```python
from build123d import *

# Parameters (mm, degrees)
SKETCH5_W           = 31
SKETCH5_H           = 31
BOSS_EXTRUDE2_DEPTH = 50
SKETCH6_W           = 5
SKETCH6_H           = 16
CUT_EXTRUDE1_DEPTH  = 50
CIRPATTERN1_COUNT   = 4
SKETCH7_R           = 5.164102758
CUT_EXTRUDE2_DEPTH  = 50
CIRPATTERN2_COUNT   = 4
FILLET1_R           = 1.5
SKETCH8_R           = 4.25
CUT_EXTRUDE3_DEPTH  = 1.5


with BuildPart() as part:
    # Sketch5 → Boss-Extrude2 (new body)
    with BuildSketch(Plane(origin=(0, 3, 0), x_dir=(1, 0, 0), z_dir=(0, 1, 0))):
        Rectangle(SKETCH5_W, SKETCH5_H)
    extrude(amount=BOSS_EXTRUDE2_DEPTH)

    # Sketch6 → Cut-Extrude1 (cut)
    with BuildSketch(Plane(origin=(0, 53, 0), x_dir=(1, 0, 0), z_dir=(0, 1, 0))):
        with Locations((-13, 0)):
            Rectangle(SKETCH6_W, SKETCH6_H)
    cut_extrude1 = extrude(amount=-CUT_EXTRUDE1_DEPTH, mode=Mode.SUBTRACT)

    # CirPattern1: Cut-Extrude1 ×4 about axis
    cirpattern1_axis = Axis((0, 0, 0), (0, 1, 0))
    for i in range(1, CIRPATTERN1_COUNT):
        add(cut_extrude1.rotate(cirpattern1_axis, i * 360 / CIRPATTERN1_COUNT), mode=Mode.SUBTRACT)

    # Sketch7 → Cut-Extrude2 (cut)
    with BuildSketch(Plane(origin=(0, 53, 0), x_dir=(1, 0, 0), z_dir=(0, 1, 0))):
        with Locations((-15.5, -15.5)):
            Circle(SKETCH7_R)
    cut_extrude2 = extrude(amount=-CUT_EXTRUDE2_DEPTH, mode=Mode.SUBTRACT)

    # CirPattern2: Cut-Extrude2 ×4 about axis
    cirpattern2_axis = Axis((0, 0, 0), (0, 1, 0))
    for i in range(1, CIRPATTERN2_COUNT):
        add(cut_extrude2.rotate(cirpattern2_axis, i * 360 / CIRPATTERN2_COUNT), mode=Mode.SUBTRACT)

    # Fillet1
    fillet1_edges = [part.edges().sort_by_distance(p)[0] for p in [
        (15.5, 28, -10.335897242),
        (10.335897242, 28, -15.5),
        (-10.335897242, 28, -15.5),
        (-15.5, 28, -10.335897242),
        (-15.5, 28, 10.335897242),
        (-10.335897242, 28, 15.5),
        (10.335897242, 28, 15.5),
        (15.5, 28, 10.335897242),
    ]]
    fillet(fillet1_edges, radius=FILLET1_R)

    # Sketch8 → Cut-Extrude3 (cut)
    with BuildSketch(Plane.XZ.offset(-3)):
        with Locations(Location((0, 0, 0), (0, 0, 270))):
            Circle(SKETCH8_R)
    extrude(amount=-CUT_EXTRUDE3_DEPTH, mode=Mode.SUBTRACT)


solid = part.part
```
Check sheet for the modelled part. Datum: model origin and axes. Units: mm. A direction names the side the tool comes from. Give positions to 0.01 mm unless a question says otherwise; leave off trailing zeros. Loops run counter-clockwise (first coordinate to the right, second up) from the corner with the lowest first, then second, coordinate; pieces in that order, holes last. Notation, with made-up numbers: M -32.5,20.5 L 1.5,20.5 A24 cw 1.5,31.5 Z; hole C 85,29 d9. An arc over 180 degrees is marked long. Answer in a Markdown table with one row per item.
1) Mould release check, pull along X, two halves, no side actions. Record for faces 1 (the face through (0, 28, -10.5)), 2 (the face through (15.5, 27.6, 8.5)), 3 (the face through (-15.18, 27.65, -9.93)), 4 (the face through (-13, 28, -8)): released by +X, released by -X, zero draft, split by the parting line, or undercut.
Solutions:
| item | result |
|---|---|
| face 1 | undercut |
| face 2 | released by +X |
| face 3 | released by -X |
| face 4 | zero draft |
2) Cross-section at B-B (z = 13.5). Enter the section's corners in (x, y).
Solutions:
| item | result |
|---|---|
| outline | M -10.74,3 L -8,3 L -8,53 L -10.74,53 Z; M 8,3 L 10.74,3 L 10.74,53 L 8,53 Z |
3) Depth check by flat-ended pin: pin 1 (1.5 mm diameter, centred on x = 12, y = 24.5, fed in from +Z); pin 2 (1.5 mm diameter, centred on x = 14, y = 19, fed in from -Z); pin 3 (5 mm diameter, centred on y = 16, z = -1.5, fed in from +X). Enter the tip coordinate at first touch or a pass-through.
Solutions:
| item | result |
|---|---|
| pin 1 | stops at z = 12.57 |
| pin 2 | stops at z = -10.85 |
| pin 3 | stops at x = 10.5 |
4) Cross-section at A-A (x = 0). Enter the section's corners in (y, z).
Solutions:
| item | result |
|---|---|
| outline | M 3,-10.5 L 53,-10.5 L 53,10.5 L 3,10.5 L 3,4.25 L 4.5,4.25 L 4.5,-4.25 L 3,-4.25 Z |
5) Thickness scan on line 1 (X direction, y = 3.75, z = 0); line 2 (X direction, y = 31, z = -7.5); line 3 (X direction, y = 36.5, z = 11.5). Record the ranges inside material, lowest first.
Solutions:
| item | result |
|---|---|
| line 1 | x = -10.5 to -4.25, 4.25 to 10.5 |
| line 2 | x = -10.5 to 10.5 |
| line 3 | x = -12.23 to -8, 8 to 12.23 |
6) Tool access check on faces 5 (the face through (-8, 28, -13)), 6 (the face through (0, 4.5, 0)), 7 (the face through (10.5, 28, 0)). Record the directions out of +Z, -Z, +X, -X, +Y, -Y that give a thin tool (end or side, any length) a straight path to the whole face; none if there is none.
Solutions:
| item | result |
|---|---|
| face 5 | -Z, +Y, -Y |
| face 6 | -Y |
| face 7 | +X, +Y, -Y |
7) Cross-section at D-D (z = 0). Enter the section's corners in (x, y).
Solutions:
| item | result |
|---|---|
| outline | M -10.5,3 L -4.25,3 L -4.25,4.5 L 4.25,4.5 L 4.25,3 L 10.5,3 L 10.5,53 L -10.5,53 Z |
